```python
from build123d import *

# Parameters (mm, degrees)
BOSS_EXTRUDE1_DEPTH = 40
SKETCH7_W           = 40
SKETCH7_H           = 10
BOSS_EXTRUDE2_DEPTH = 2
SKETCH8_R           = 2.05
CUT_EXTRUDE1_DEPTH  = 38


with BuildPart() as part:
    # Sketch6 → Boss-Extrude1 (new body)
    with BuildSketch(Plane(origin=(0, 0, 0), x_dir=(1, 0, 0), z_dir=(0, 1, 0))):
        with BuildLine():
            Line((20, 28.809017417), (-20, 28.809017417))
            Line((-20, 28.809017417), (-20, 15))
            ThreePointArc((-20, 15), (0, 25), (20, 15))
            Line((20, 15), (20, 28.809017417))
        make_face()
    extrude(amount=BOSS_EXTRUDE1_DEPTH)

    # Sketch7 → Boss-Extrude2 (add)
    with BuildSketch(Plane(origin=(0, 5, 0), x_dir=(-1, 0, 0), z_dir=(0, -1, 0))):
        with Locations((0, 21.508861193)):
            Rectangle(SKETCH7_W, SKETCH7_H)
    extrude(amount=BOSS_EXTRUDE2_DEPTH)

    # Sketch8 → Cut-Extrude1 (cut, through all)
    with BuildSketch(Plane.XZ.offset(-3)):
        with Locations((0, -20)):
            Circle(SKETCH8_R)
    extrude(amount=-CUT_EXTRUDE1_DEPTH, mode=Mode.SUBTRACT)


solid = part.part
```
The model under review builds one solid part; all positions refer to its coordinate system, in mm. A direction names the side the tool comes from. Give positions to 0.01 mm unless a question says otherwise; leave off trailing zeros. Write each loop counter-clockwise with the first axis right and the second up, starting at its lowest first coordinate (ties: lowest second). Pieces come first, ordered by that corner, then holes. Notation, with made-up numbers: M 13,56 L 49,56 A25 ccw 49,70 Z; hole C 29,37 d4. An arc over 180 degrees is marked long. Write each question's results on one line, items separated by ' | '. Start each with the question number.
1. We need section B-B (z = -20). Write out the cut boundary in (x, y).
2. Insertion check: pin 1 Ø0.6 at (x, y) = (-7.5, 4) entering from +Z; pin 2 Ø6 at (x, y) = (-14, 16) entering from +Z; pin 3 Ø2 at (x, z) = (-10, -21.5) entering from -Y. Each pin has a flat end and moves straight along its axis. Give the tip position at first contact, or say it passes through.
3. Mouldability with a two-part tool opening along X and no side actions: class faces 1 (the flat face through (0, 20, -28.809)), 2 (the flat face through (20, 20, -22)), 3 (the flat face through (0, 3, -23)) as released by +X, released by -X, zero draft, split by the parting line, or undercut.
4. For faces 4 (the cylindrical face through (-1.5, 4, -18.6)), 5 (the flat face through (0, 5, -23)), 6 (the flat face through (0, 4, -16.509)), list the 3-axis set-ups (+Z, -Z, +X, -X, +Y, -Y) from which the entire face can be reached by the end or side of a thin tool; tool diameter is ignored.
5. We need section D-D (x = -10.5). Write out the cut boundary in (y, z), and give its area (3 significant figures).
6. We need section C-C (y = 3.5). Write out the cut boundary in (x, z).
7. For probe 1 along Z at (x, y) = (0, 3.8); probe 2 along Y at (x, z) = (13.5, -17.5); probe 3 along X at (y, z) = (2.5, -20.25), list the stretches that pass through material, from the lowest coordinate up. Write a range as [from, to].
8. We need section A-A (x = 0). Write out the cut boundary in (y, z).
Results found:
1) outline: M -20,0 L -15,0 L -15,3 L -2.05,3 L -2.05,5 L -15,5 L -15,40 L -20,40 Z; M 2.05,3 L 15,3 L 15,0 L 20,0 L 20,40 L 15,40 L 15,5 L 2.05,5 Z
2) pin 1: stops at z = -16.51 | pin 2: stops at z = -18.33 | pin 3: stops at y = 3
3) face 1: zero draft | face 2: released by +X | face 3: undercut
4) face 4: +Y, -Y | face 5: +Z, +Y | face 6: +Z, +Y, -Y
5) outline: M 0,-28.81 L 40,-28.81 L 40,-22.69 L 5,-22.69 L 5,-16.51 L 3,-16.51 L 3,-22.69 L 0,-22.69 Z | area: 257 mm^2
6) outline: M -20,-28.81 L 20,-28.81 L 20,-15 A25 cw 18.77,-16.51 L -18.77,-16.51 A25 cw -20,-15 Z; hole C 0,-20 d4.1
7) probe 1: z = [-28.81, -22.05], [-17.95, -16.51] | probe 2: y = [3, 5] | probe 3: x = [-20, -14.66], [14.66, 20]
8) outline: M 0,-28.81 L 40,-28.81 L 40,-25 L 5,-25 L 5,-22.05 L 3,-22.05 L 3,-25 L 0,-25 Z; M 3,-17.95 L 5,-17.95 L 5,-16.51 L 3,-16.51 Z
